For this review, take the finished solid that the model builds, in its own axes (mm). Face numbers are marked on the shaded views. A direction names the side the tool comes from. Round coordinates to 2 decimals unless told otherwise and drop trailing zeros. Loops run counter-clockwise (first coordinate to the right, second up) from the corner with the lowest first, then second, coordinate; pieces in that order, holes last. Notation, with made-up numbers: M -35.5,2.25 L 23.5,2.25 A24 ccw 23.5,19.25 Z; hole C 8,34.5 d2. An arc over 180 degrees is marked long. One line per question, with ' | ' between items. Start each with the question number.
1) For probe 1 along Z at (x, y) = (0, 1.6); probe 2 along Y at (x, z) = (-2.25, -0.5), list the stretches that pass through material, from the lowest coordinate up. Write a range as from..to.
2) We need section B-B (y = 6.75). Give the boundary of the cut face in (x, z).
3) For pin 1 Ø1 at (y, z) = (5.5, -2.5) entering from -X; pin 2 Ø1.5 at (y, z) = (6, 1) entering from +X; pin 3 Ø1.1 at (x, y) = (1, 5) entering from -Z, all flat-tipped, find the tip position at first contact; note any pin that passes through.
4) We need section A-A (x = 0). Give the boundary of the cut face in (y, z).
5) We need section C-C (y = 1.25). Give the boundary of the cut face in (x, z), and give its area (3 significant figures).
6) Mouldability with a two-part tool opening along X and no side actions: class the marked faces 1, 2 and 3 as pulls with the +X half, pulls with the -X half, needs draft (parallel to the pull), parting line crosses it, or undercut.
7) For the marked faces 4 and 5, list the 3-axis set-ups (+Z, -Z, +X, -X, +Y, -Y) from which the entire face can be reached by the end or side of a thin tool; tool diameter is ignored.
```python
from build123d import *

# Parameters (mm, degrees)
CUT_EXTRUDE1_DEPTH = 3.81


with BuildPart() as part:
    # Sketch1 → Revolve1 (revolve)
    with BuildSketch(Plane.XY):
        with BuildLine():
            Line((-1.4732, 0), (-8.128, 0))
            Line((-8.128, 0), (-8.128, 2.032))
            Line((-8.128, 2.032), (-7.034252752, 6.1139203))
            ThreePointArc((-7.034252752, 6.1139203), (-6.308494697, 7.200093987), (-5.071491473, 7.62))
            Line((-5.071491473, 7.62), (-1.4732, 7.62))
            Line((-1.4732, 7.62), (-1.4732, 0))
        make_face()
    revolve(axis=Axis((0, 0, 0), (0, -1, 0)))

    # Sketch2 → Cut-Extrude1 (cut)
    with BuildSketch(Plane(origin=(0, 7.62, 0), x_dir=(1, 0, 0), z_dir=(0, 1, 0))):
        Polygon((-4.839349956, 0), (-2.419674978, -4.191), (2.419674978, -4.191), (4.839349956, 0), (2.419674978, 4.191), (-2.419674978, 4.191), align=None)
    extrude(amount=-CUT_EXTRUDE1_DEPTH, mode=Mode.SUBTRACT)


solid = part.part
```
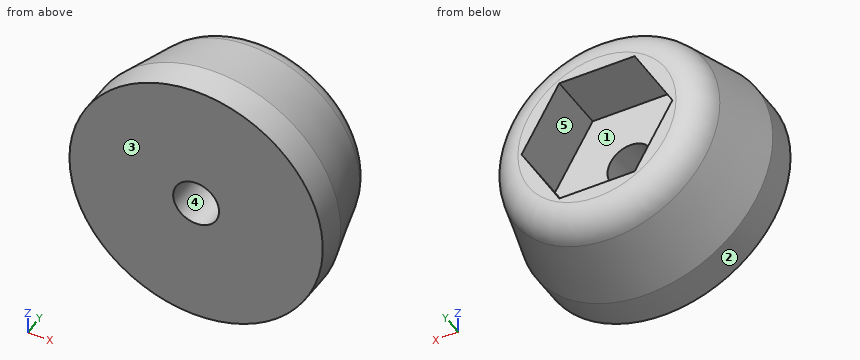
Answers below:
1) probe 1: -8.13..-1.47, 1.47..8.13 | probe 2: 0..3.81
2) outline: C 0,0 d13.48; hole M -4.84,0 L -2.42,-4.19 L 2.42,-4.19 L 4.84,0 L 2.42,4.19 L -2.42,4.19 Z
3) pin 1: x = -6.97 | pin 2: x = 7.22 | pin 3: z = -7.43
4) outline: M 0,-8.13 L 2.03,-8.13 L 6.11,-7.03 A2.03 ccw 7.62,-5.07 L 7.62,-4.19 L 3.81,-4.19 L 3.81,-1.47 L 0,-1.47 Z; M 0,1.47 L 3.81,1.47 L 3.81,4.19 L 7.62,4.19 L 7.62,5.07 A2.03 ccw 6.11,7.03 L 2.03,8.13 L 0,8.13 Z
5) outline: C 0,0 d16.26; hole C 0,0 d2.95 | area: 201 mm^2
6) face 1: undercut | face 2: parting line crosses it | face 3: needs draft
7) face 4: +Y, -Y | face 5: +Y
